Job drawing, mm, ordinate dimensions from the low corner. One solid piece. A direction names the side the tool comes from. Coordinates: 2 decimals unless noted, no trailing zeros. Write each loop counter-clockwise with the first axis right and the second up, starting at its lowest first coordinate (ties: lowest second). Pieces come first, ordered by that corner, then holes. Notation, with made-up numbers: (33.25, 80) -> (77.25, 80) arc R20 ccw to (77.25, 96) -> close; hole circle Ø9 at (49, 50.5). An arc over 180 degrees is marked (long way). One line per question, with ' | ' between items. Start each with the question number.
Item 1: 3-axis set-ups, long thin cutter, end or side, ignore diameter. For the marked faces 1 and 2: which of +Z, -Z, +X, -X, +Y, -Y reach the whole face in a straight line?
Item 2: Saw through at B-B (y = 77). List the corners of the cut face in (x, z).
Item 3: Pin check, flat tips, straight feed: pin 1 (1.5 mm diameter, centred on x = 33, z = 4, fed in from +Y); pin 2 (2.5 mm diameter, centred on y = 76.5, z = 6.5, fed in from -X); pin 3 (4 mm diameter, centred on x = 38.6, z = 6, fed in from +Y); pin 4 (5 mm diameter, centred on x = 54.5, z = 7, fed in from -Y). Stop position of each tip, or through.
Item 4: Probe probe 1 along X at (y, z) = (11.25, 6) (1 decimal); probe 2 along Y at (x, z) = (8.5, 4.75) (1 decimal); probe 3 along Z at (x, y) = (8, 111). List the from-to ranges inside material, lowest first. Write a range as [from, to].
Item 5: Saw through at D-D (y = 11.5). List the corners of the cut face in (x, z) (1 decimal).
Item 6: Saw through at C-C (x = 25). List the corners of the cut face in (y, z), and give its area (3 significant figures).
Item 7: Saw through at A-A (z = 10.5). List the corners of the cut face in (x, y) (1 decimal), and give its area (3 significant figures).
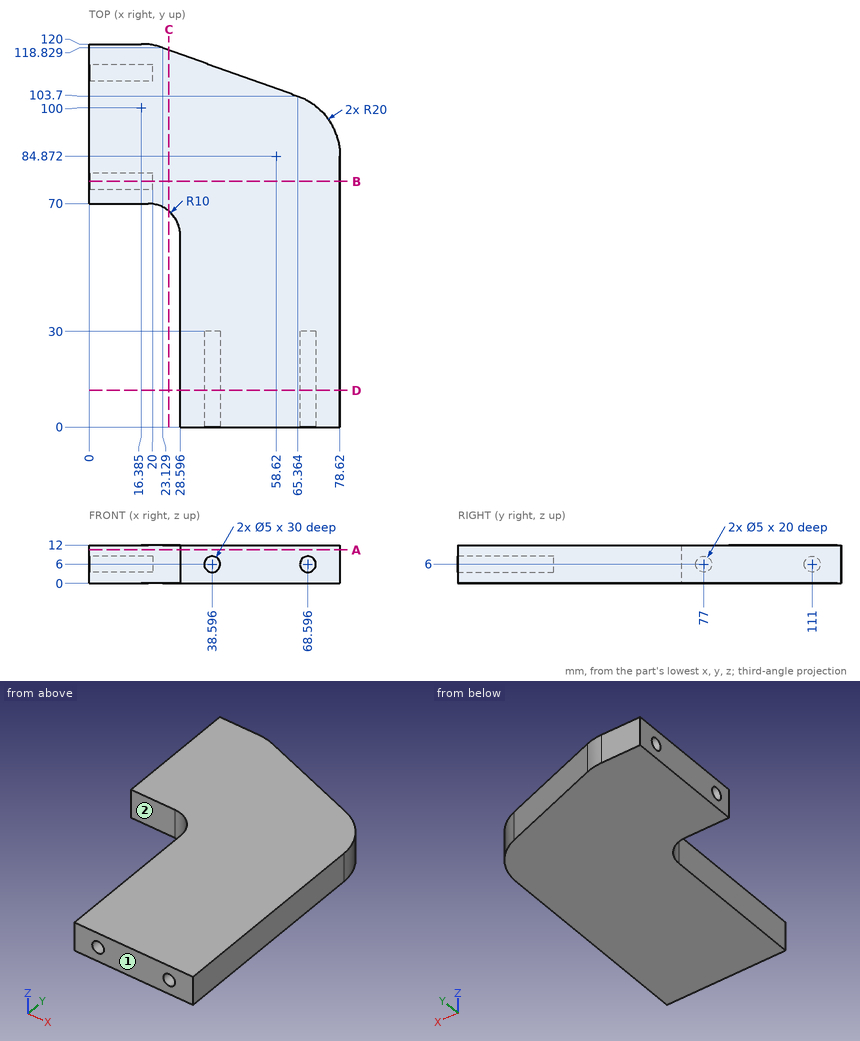
From the geometry:
1) face 1: +Z, -Z, +X, -X, -Y | face 2: +Z, -Z, -X, -Y
2) outline: (0, 0) -> (78.62, 0) -> (78.62, 12) -> (0, 12) -> (0, 8.5) -> (20, 8.5) -> (20, 3.5) -> (0, 3.5) -> close
3) pin 1: y = 115.56 | pin 2: x = 20 | pin 3: y = 114 | pin 4: y = 0
4) probe 1: [28.6, 36.1], [41.1, 66.1], [71.1, 78.6] | probe 2: [70, 74.8], [79.2, 108.8], [113.2, 120] | probe 3: [0, 3.5], [8.5, 12]
5) outline: (28.6, 0) -> (78.6, 0) -> (78.6, 12) -> (28.6, 12) -> close; hole circle Ø5 at (38.6, 6); hole circle Ø5 at (68.6, 6)
6) outline: (67.68, 0) -> (118.16, 0) -> (118.16, 12) -> (67.68, 12) -> close | area: 606 mm2
7) outline: (0, 70) -> (18.6, 70) arc R10 cw to (28.6, 60) -> (28.6, 0) -> (78.6, 0) -> (78.6, 84.9) arc R20 ccw to (65.4, 103.7) -> (23.1, 118.8) arc R20 ccw to (16.4, 120) -> (0, 120) -> close | area: 6,800 mm2
